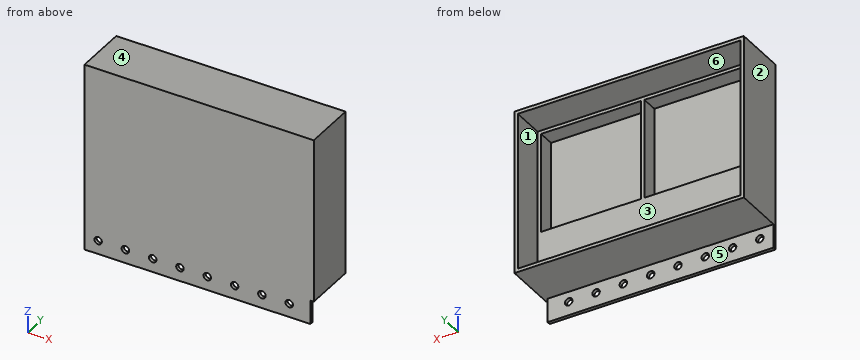
```python
from build123d import *

# Parameters (mm, degrees)
SKETCH1_W            = 609.6
SKETCH1_H            = 304.8
SKETCH1_W_2          = 93
SKETCH1_H_2          = 93
BOSS_EXTRUDE1_DEPTH  = 15.24
SKETCH2_W            = 609.6
SKETCH2_H            = 304.8
BOSS_EXTRUDE2_DEPTH  = 3.175
SKETCH3_W            = 609.6
SKETCH3_H            = 304.8
SKETCH3_W_2          = 603.25
SKETCH3_H_2          = 254
BOSS_EXTRUDE3_DEPTH  = 30.48
SKETCH4_OUTSIDE_W    = 748.262
SKETCH4_OUTSIDE_H    = 443.462
SKETCH4_OUTSIDE_W_2  = 609.6
SKETCH4_OUTSIDE_H_2  = 260.35
CUT_EXTRUDE1_DEPTH   = 45.72
SKETCH5_R            = 3.4925
CUT_EXTRUDE2_DEPTH   = 344.830071983
SKETCH6_W            = 327.140785269
SKETCH6_H            = 256.091806272
TEMPORARY_CUT_DEPTH  = 430.914472374
SKETCH7_W            = 260.35
SKETCH7_H            = 48.895
TEMPORARY_SIDE_DEPTH = 3.175
SKETCH8_W            = 381.398207811
SKETCH8_H            = 265.653299783
CUT_EXTRUDE3_DEPTH   = 354.138073599
SKETCH9_W            = 213.3875
SKETCH9_H            = 48.895
BOSS_EXTRUDE4_DEPTH  = 3.175


with BuildPart() as part:
    # Sketch1 → Boss-Extrude1 (new body)
    with BuildSketch(Plane(origin=(0, 0, 0), x_dir=(1, 0, 0), z_dir=(0, 1, 0))):
        Rectangle(SKETCH1_W, SKETCH1_H)
        with Locations((-48.0875, 29.7)):
            Rectangle(SKETCH1_W_2, SKETCH1_H_2, mode=Mode.SUBTRACT)
        with Locations((-144.2625, 29.7)):
            Rectangle(SKETCH1_W_2, SKETCH1_H_2, mode=Mode.SUBTRACT)
        with Locations((-144.2625, -66.475)):
            Rectangle(SKETCH1_W_2, SKETCH1_H_2, mode=Mode.SUBTRACT)
        with Locations((-48.0875, -66.475)):
            Rectangle(SKETCH1_W_2, SKETCH1_H_2, mode=Mode.SUBTRACT)
        with Locations((-240.4375, 29.7)):
            Rectangle(SKETCH1_W_2, SKETCH1_H_2, mode=Mode.SUBTRACT)
        with Locations((-240.4375, -66.475)):
            Rectangle(SKETCH1_W_2, SKETCH1_H_2, mode=Mode.SUBTRACT)
        with Locations((48.0875, 29.7)):
            Rectangle(SKETCH1_W_2, SKETCH1_H_2, mode=Mode.SUBTRACT)
        with Locations((48.0875, -66.475)):
            Rectangle(SKETCH1_W_2, SKETCH1_H_2, mode=Mode.SUBTRACT)
        with Locations((144.2625, 29.7)):
            Rectangle(SKETCH1_W_2, SKETCH1_H_2, mode=Mode.SUBTRACT)
        with Locations((144.2625, -66.475)):
            Rectangle(SKETCH1_W_2, SKETCH1_H_2, mode=Mode.SUBTRACT)
        with Locations((240.4375, 29.7)):
            Rectangle(SKETCH1_W_2, SKETCH1_H_2, mode=Mode.SUBTRACT)
        with Locations((240.4375, -66.475)):
            Rectangle(SKETCH1_W_2, SKETCH1_H_2, mode=Mode.SUBTRACT)
    extrude(amount=BOSS_EXTRUDE1_DEPTH)

    # Sketch2 → Boss-Extrude2 (add)
    with BuildSketch(Plane(origin=(0, 0, 0), x_dir=(-1, 0, 0), z_dir=(0, -1, 0))):
        Rectangle(SKETCH2_W, SKETCH2_H)
    extrude(amount=BOSS_EXTRUDE2_DEPTH)

    # Sketch3 → Boss-Extrude3 (add)
    with BuildSketch(Plane(origin=(0, 15.24, 0), x_dir=(1, 0, 0), z_dir=(0, 1, 0))):
        Rectangle(SKETCH3_W, SKETCH3_H)
        Rectangle(SKETCH3_W_2, SKETCH3_H_2, mode=Mode.SUBTRACT)
    extrude(amount=BOSS_EXTRUDE3_DEPTH)

    # Sketch4 outside → Cut-Extrude1 (cut)
    with BuildSketch(Plane(origin=(0, 45.72, 0), x_dir=(1, 0, 0), z_dir=(0, 1, 0))):
        Rectangle(SKETCH4_OUTSIDE_W, SKETCH4_OUTSIDE_H)
        Rectangle(SKETCH4_OUTSIDE_W_2, SKETCH4_OUTSIDE_H_2, mode=Mode.SUBTRACT)
    extrude(amount=-CUT_EXTRUDE1_DEPTH, mode=Mode.SUBTRACT)

    # Sketch5 → Cut-Extrude2 (cut, through all)
    with BuildSketch(Plane(origin=(0, 0, 0), x_dir=(1, 0, 0), z_dir=(0, 1, 0))):
        with Locations(Location((-292.1, -139.7, 0), (0, 0, 270))):
            Circle(SKETCH5_R)
        with Locations(Location((-266.7, -139.7, 0), (0, 0, 270))):
            Circle(SKETCH5_R)
        with Locations(Location((-241.3, -139.7, 0), (0, 0, 270))):
            Circle(SKETCH5_R)
        with Locations(Location((-215.9, -139.7, 0), (0, 0, 270))):
            Circle(SKETCH5_R)
        with Locations(Location((-190.5, -139.7, 0), (0, 0, 270))):
            Circle(SKETCH5_R)
        with Locations(Location((-165.1, -139.7, 0), (0, 0, 270))):
            Circle(SKETCH5_R)
        with Locations(Location((-139.7, -139.7, 0), (0, 0, 270))):
            Circle(SKETCH5_R)
        with Locations(Location((-114.3, -139.7, 0), (0, 0, 270))):
            Circle(SKETCH5_R)
        with Locations(Location((-88.9, -139.7, 0), (0, 0, 270))):
            Circle(SKETCH5_R)
        with Locations(Location((-63.5, -139.7, 0), (0, 0, 270))):
            Circle(SKETCH5_R)
        with Locations(Location((-38.1, -139.7, 0), (0, 0, 270))):
            Circle(SKETCH5_R)
        with Locations(Location((-12.7, -139.7, 0), (0, 0, 270))):
            Circle(SKETCH5_R)
        with Locations(Location((12.7, 139.7, 0), (0, 0, 270))):
            Circle(SKETCH5_R)
        with Locations(Location((38.1, 139.7, 0), (0, 0, 270))):
            Circle(SKETCH5_R)
        with Locations(Location((63.5, 139.7, 0), (0, 0, 270))):
            Circle(SKETCH5_R)
        with Locations(Location((88.9, 139.7, 0), (0, 0, 270))):
            Circle(SKETCH5_R)
        with Locations(Location((114.3, 139.7, 0), (0, 0, 270))):
            Circle(SKETCH5_R)
        with Locations(Location((139.7, 139.7, 0), (0, 0, 270))):
            Circle(SKETCH5_R)
        with Locations(Location((165.1, 139.7, 0), (0, 0, 270))):
            Circle(SKETCH5_R)
        with Locations(Location((190.5, 139.7, 0), (0, 0, 270))):
            Circle(SKETCH5_R)
        with Locations(Location((215.9, 139.7, 0), (0, 0, 270))):
            Circle(SKETCH5_R)
        with Locations(Location((241.3, 139.7, 0), (0, 0, 270))):
            Circle(SKETCH5_R)
        with Locations(Location((-292.1, 139.7, 0), (0, 0, 270))):
            Circle(SKETCH5_R)
        with Locations(Location((-266.7, 139.7, 0), (0, 0, 270))):
            Circle(SKETCH5_R)
        with Locations(Location((-241.3, 139.7, 0), (0, 0, 270))):
            Circle(SKETCH5_R)
        with Locations(Location((-215.9, 139.7, 0), (0, 0, 270))):
            Circle(SKETCH5_R)
        with Locations(Location((-190.5, 139.7, 0), (0, 0, 270))):
            Circle(SKETCH5_R)
        with Locations(Location((-165.1, 139.7, 0), (0, 0, 270))):
            Circle(SKETCH5_R)
        with Locations(Location((-139.7, 139.7, 0), (0, 0, 270))):
            Circle(SKETCH5_R)
        with Locations(Location((-114.3, 139.7, 0), (0, 0, 270))):
            Circle(SKETCH5_R)
        with Locations(Location((-88.9, 139.7, 0), (0, 0, 270))):
            Circle(SKETCH5_R)
        with Locations(Location((-63.5, 139.7, 0), (0, 0, 270))):
            Circle(SKETCH5_R)
        with Locations(Location((-38.1, 139.7, 0), (0, 0, 270))):
            Circle(SKETCH5_R)
        with Locations(Location((-12.7, 139.7, 0), (0, 0, 270))):
            Circle(SKETCH5_R)
        with Locations(Location((266.7, 139.7, 0), (0, 0, 270))):
            Circle(SKETCH5_R)
        with Locations(Location((292.1, 139.7, 0), (0, 0, 270))):
            Circle(SKETCH5_R)
        with Locations(Location((12.7, -139.7, 0), (0, 0, 270))):
            Circle(SKETCH5_R)
        with Locations(Location((38.1, -139.7, 0), (0, 0, 270))):
            Circle(SKETCH5_R)
        with Locations(Location((63.5, -139.7, 0), (0, 0, 270))):
            Circle(SKETCH5_R)
        with Locations(Location((88.9, -139.7, 0), (0, 0, 270))):
            Circle(SKETCH5_R)
        with Locations(Location((114.3, -139.7, 0), (0, 0, 270))):
            Circle(SKETCH5_R)
        with Locations(Location((139.7, -139.7, 0), (0, 0, 270))):
            Circle(SKETCH5_R)
        with Locations(Location((165.1, -139.7, 0), (0, 0, 270))):
            Circle(SKETCH5_R)
        with Locations(Location((190.5, -139.7, 0), (0, 0, 270))):
            Circle(SKETCH5_R)
        with Locations(Location((215.9, -139.7, 0), (0, 0, 270))):
            Circle(SKETCH5_R)
        with Locations(Location((241.3, -139.7, 0), (0, 0, 270))):
            Circle(SKETCH5_R)
        with Locations(Location((266.7, -139.7, 0), (0, 0, 270))):
            Circle(SKETCH5_R)
        with Locations(Location((292.1, -139.7, 0), (0, 0, 270))):
            Circle(SKETCH5_R)
    extrude(amount=-CUT_EXTRUDE2_DEPTH, mode=Mode.SUBTRACT)

    # Sketch6 → Temporary_Cut (cut, through all)
    with BuildSketch(Plane(origin=(-94.5875, 0, 0), x_dir=(0, 0, -1), z_dir=(1, 0, 0))):
        with Locations((-7.828616148, 44.910513642)):
            Rectangle(SKETCH6_W, SKETCH6_H)
    extrude(amount=TEMPORARY_CUT_DEPTH, mode=Mode.SUBTRACT)

    # Sketch7 → Temporary_Side (add)
    with BuildSketch(Plane(origin=(-94.5875, 0, 0), x_dir=(0, 0, -1), z_dir=(1, 0, 0))):
        with Locations((0, 21.2725)):
            Rectangle(SKETCH7_W, SKETCH7_H)
    extrude(amount=TEMPORARY_SIDE_DEPTH)

    # Sketch8 → Cut-Extrude3 (cut, through all)
    with BuildSketch(Plane.XY.offset(19.975)):
        with Locations((-174.977799194, 15.778240494)):
            Rectangle(SKETCH8_W, SKETCH8_H)
    extrude(amount=CUT_EXTRUDE3_DEPTH, mode=Mode.SUBTRACT)

    # Sketch9 → Boss-Extrude4 (add)
    with BuildSketch(Plane.XY.offset(19.975)):
        with Locations((-198.10625, 21.2725)):
            Rectangle(SKETCH9_W, SKETCH9_H)
    extrude(amount=BOSS_EXTRUDE4_DEPTH)


solid = part.part
```
The listing builds one solid part. Answer for the finished solid, in the listing's coordinates (mm). Face numbers are marked on the shaded views. A direction names the side the tool comes from. Round coordinates to 2 decimals unless told otherwise and drop trailing zeros. Loops run counter-clockwise (first coordinate to the right, second up) from the corner with the lowest first, then second, coordinate; pieces in that order, holes last. Notation, with made-up numbers: (-23.5, -17.5) - (-2.5, -17.5) arc R27 ccw to (-2.5, -1.5) - close; hole circle Ø5 at (52.5, -28.75). An arc over 180 degrees is marked (long way). Return JSON: item names as keys, results as strings. Group by question number.
1. The part is cut by section D-D on y = 6. State how many separate pieces and enclosed holes the cut face has, then the cut area to 3 significant figures.
2. Consider probe 1 along X at (y, z) = (7, -38.5); probe 2 along X at (y, z) = (42.5, -27.5) (1 decimal); probe 3 along Z at (x, y) = (-141.5, 0.5) (3 decimals). Determine where each line is inside the solid, lowest interval first.
3. The part is cut by section C-C on z = -51. Determine the outline of the cut face in (x, y) (1 decimal), then the cut area to 3 significant figures.
4. This flat-tipped pin is pushed along its axis until it touches: P1, Ø4, axis at x = -185, y = 18.5, coming from the -Z side (3 decimals). Where does it stop, or does it pass through?
5. Which of the six approach directions +Z, -Z, +X, -X, +Y, -Y give full straight-line access (tool end or side, diameter ignored) to the marked faces 1 and 2?
6. The mould has two halves that part along Z. Classify the marked faces 3, 4, 5 and 6: pulls with the +Z half, pulls with the -Z half, needs draft (parallel to the pull), parting line crosses it, or undercut.
Resolved:
{
 "1": {"separate pieces": "1", "enclosed holes": "2", "area": "15,400 mm²"},
 "2": {"probe 1": "x = -304.8 to -286.94, -193.94 to -190.76, -97.76 to -91.41", "probe 2": "x = -304.8 to -301.6, -94.6 to -91.4", "probe 3": "z = -130.175 to -76.2, 16.8 to 23.15"},
 "3": {"outline": "(-304.8, -3.2) - (-91.4, -3.2) - (-91.4, 45.7) - (-94.6, 45.7) - (-94.6, 15.2) - (-97.8, 15.2) - (-97.8, 0) - (-190.8, 0) - (-190.8, 15.2) - (-193.9, 15.2) - (-193.9, 0) - (-286.9, 0) - (-286.9, 15.2) - (-301.6, 15.2) - (-301.6, 45.7) - (-304.8, 45.7) - close", "area": "1,290 mm²"},
 "4": {"P1": "stops at z = -130.175"},
 "5": {"face 1": "+Y", "face 2": "+Z, -Z, -X, +Y, -Y"},
 "6": {"face 3": "undercut", "face 4": "pulls with the +Z half", "face 5": "needs draft", "face 6": "undercut"}
}
